```python
from build123d import *

# Parameters (mm, degrees)
F0_R     = 1.2
F0_W     = 10.5
F0_H     = 10.5
F1_DEPTH = 1.5
F2_DEPTH = 5.25
F3_DEPTH = 5.75
F5_DEPTH = 2


# Not quite as in the source:
# - a feature names something its author has since deleted; it is built from what else it names


with BuildPart() as f1:
    # F0 (on Top) → F1 (new body)
    with BuildSketch(Plane.XY):
        with BuildLine():
            Line((14.9310000289, -10.5), (14.9310000289, 10.5))
            ThreePointArc((14.9310000289, 10.5), (13.4665339264, 14.0355339264), (9.931, 15.5000000289))
            Line((9.931, 15.5000000289), (-9.931, 15.5000000289))
            ThreePointArc((-9.931, 15.5000000289), (-13.4665339264, 14.0355339264), (-14.9310000289, 10.5))
            Line((-14.9310000289, 10.5), (-14.9310000289, -10.5))
            ThreePointArc((-14.9310000289, -10.5), (-13.4665339264, -14.0355339264), (-9.931, -15.5000000289))
            Line((-9.931, -15.5000000289), (9.931, -15.5000000289))
            ThreePointArc((9.931, -15.5000000289), (13.4665339264, -14.0355339264), (14.9310000289, -10.5))
        make_face()
        with BuildLine():
            Line((-9.931, 13.5000000289), (-7.581, 13.5000000289))
            Line((-7.581, 13.5000000289), (0.069, 13.5000000289))
            Line((0.069, 13.5000000289), (4.769, 13.5000000289))
            Line((4.769, 13.5000000289), (9.931, 13.5000000289))
            ThreePointArc((9.931, 13.5000000289), (12.052320364, 12.621320364), (12.9310000289, 10.5))
            Line((12.9310000289, 10.5), (12.9310000289, -10.5))
            ThreePointArc((12.9310000289, -10.5), (12.052320364, -12.621320364), (9.931, -13.5000000289))
            Line((9.931, -13.5000000289), (4.769, -13.5000000289))
            Line((4.769, -13.5000000289), (0.069, -13.5000000289))
            Line((0.069, -13.5000000289), (-7.581, -13.5000000289))
            Line((-7.581, -13.5000000289), (-9.931, -13.5000000289))
            ThreePointArc((-9.931, -13.5000000289), (-12.052320364, -12.621320364), (-12.9310000289, -10.5))
            Line((-12.9310000289, -10.5), (-12.9310000289, -8.1))
            Line((-12.9310000289, -8.1), (-12.9310000289, 8.1))
            Line((-12.9310000289, 8.1), (-12.9310000289, 10.5))
            ThreePointArc((-12.9310000289, 10.5), (-12.052320364, 12.621320364), (-9.931, 13.5000000289))
        make_face(mode=Mode.SUBTRACT)
        with BuildLine():
            ThreePointArc((4.769, -10.45), (2.419, -8.1), (0.069, -10.45))
            ThreePointArc((0.069, -10.45), (2.419, -12.8), (4.769, -10.45))
        make_face()
        with Locations((2.419, -10.45)):
            Circle(F0_R, mode=Mode.SUBTRACT)
        with BuildLine():
            ThreePointArc((4.769, 10.45), (2.419, 12.8), (0.069, 10.45))
            ThreePointArc((0.069, 10.45), (2.419, 8.1), (4.769, 10.45))
        make_face()
        with Locations((2.419, 10.45)):
            Circle(F0_R, mode=Mode.SUBTRACT)
        with BuildLine():
            ThreePointArc((-9.931, 8.1), (-11.5927009358, 12.1117009358), (-7.581, 10.45))
            Line((-7.581, 10.45), (-7.581, 13.5000000289))
            Line((-7.581, 13.5000000289), (-9.931, 13.5000000289))
            ThreePointArc((-9.931, 13.5000000289), (-12.052320364, 12.621320364), (-12.9310000289, 10.5))
            Line((-12.9310000289, 10.5), (-12.9310000289, 8.1))
            Line((-12.9310000289, 8.1), (-9.931, 8.1))
        make_face()
        with BuildLine():
            Line((-9.931, -8.1), (-12.9310000289, -8.1))
            Line((-12.9310000289, -8.1), (-12.9310000289, -10.5))
            ThreePointArc((-12.9310000289, -10.5), (-12.052320364, -12.621320364), (-9.931, -13.5000000289))
            Line((-9.931, -13.5000000289), (-7.581, -13.5000000289))
            Line((-7.581, -13.5000000289), (-7.581, -10.45))
            ThreePointArc((-7.581, -10.45), (-11.5927009358, -12.1117009358), (-9.931, -8.1))
        make_face()
        with BuildLine():
            Line((-7.581, 13.5000000289), (-7.581, 10.45))
            ThreePointArc((-7.581, 10.45), (-8.2692990642, 8.7882990642), (-9.931, 8.1))
            Line((-9.931, 8.1), (-12.9310000289, 8.1))
            Line((-12.9310000289, 8.1), (-12.9310000289, -8.1))
            Line((-12.9310000289, -8.1), (-9.931, -8.1))
            ThreePointArc((-9.931, -8.1), (-8.2692990642, -8.7882990642), (-7.581, -10.45))
            Line((-7.581, -10.45), (-7.581, -13.5000000289))
            Line((-7.581, -13.5000000289), (0.069, -13.5000000289))
            Line((0.069, -13.5000000289), (0.069, -10.45))
            ThreePointArc((0.069, -10.45), (2.419, -8.1), (4.769, -10.45))
            Line((4.769, -10.45), (4.769, -13.5000000289))
            Line((4.769, -13.5000000289), (9.931, -13.5000000289))
            ThreePointArc((9.931, -13.5000000289), (12.052320364, -12.621320364), (12.9310000289, -10.5))
            Line((12.9310000289, -10.5), (12.9310000289, 10.5))
            ThreePointArc((12.9310000289, 10.5), (12.052320364, 12.621320364), (9.931, 13.5000000289))
            Line((9.931, 13.5000000289), (4.769, 13.5000000289))
            Line((4.769, 13.5000000289), (4.769, 10.45))
            ThreePointArc((4.769, 10.45), (2.419, 8.1), (0.069, 10.45))
            Line((0.069, 10.45), (0.069, 13.5000000289))
            Line((0.069, 13.5000000289), (-7.581, 13.5000000289))
        make_face()
        with Locations((2.469, 0)):
            Rectangle(F0_W, F0_H, mode=Mode.SUBTRACT)
        with BuildLine():
            ThreePointArc((-7.581, -10.45), (-8.2692990642, -8.7882990642), (-9.931, -8.1))
            ThreePointArc((-9.931, -8.1), (-11.5927009358, -12.1117009358), (-7.581, -10.45))
        make_face()
        with Locations((-9.931, -10.45)):
            Circle(F0_R, mode=Mode.SUBTRACT)
        with BuildLine():
            Line((0.069, -10.45), (0.069, -13.5000000289))
            Line((0.069, -13.5000000289), (4.769, -13.5000000289))
            Line((4.769, -13.5000000289), (4.769, -10.45))
            ThreePointArc((4.769, -10.45), (2.419, -12.8), (0.069, -10.45))
        make_face()
        with BuildLine():
            ThreePointArc((-9.931, 8.1), (-8.2692990642, 8.7882990642), (-7.581, 10.45))
            ThreePointArc((-7.581, 10.45), (-11.5927009358, 12.1117009358), (-9.931, 8.1))
        make_face()
        with Locations((-9.931, 10.45)):
            Circle(F0_R, mode=Mode.SUBTRACT)
        with BuildLine():
            Line((4.769, 13.5000000289), (0.069, 13.5000000289))
            Line((0.069, 13.5000000289), (0.069, 10.45))
            ThreePointArc((0.069, 10.45), (2.419, 12.8), (4.769, 10.45))
            Line((4.769, 10.45), (4.769, 13.5000000289))
        make_face()
    extrude(amount=F1_DEPTH)

    # F0 (on Top) → F2 (join)
    with BuildSketch(Plane.XY):
        with BuildLine():
            ThreePointArc((-9.931, 8.1), (-11.5927009358, 12.1117009358), (-7.581, 10.45))
            Line((-7.581, 10.45), (-7.581, 13.5000000289))
            Line((-7.581, 13.5000000289), (-9.931, 13.5000000289))
            ThreePointArc((-9.931, 13.5000000289), (-12.052320364, 12.621320364), (-12.9310000289, 10.5))
            Line((-12.9310000289, 10.5), (-12.9310000289, 8.1))
            Line((-12.9310000289, 8.1), (-9.931, 8.1))
        make_face()
        with BuildLine():
            ThreePointArc((-9.931, 8.1), (-8.2692990642, 8.7882990642), (-7.581, 10.45))
            ThreePointArc((-7.581, 10.45), (-11.5927009358, 12.1117009358), (-9.931, 8.1))
        make_face()
        with Locations((-9.931, 10.45)):
            Circle(F0_R, mode=Mode.SUBTRACT)
        with BuildLine():
            ThreePointArc((4.769, 10.45), (2.419, 12.8), (0.069, 10.45))
            ThreePointArc((0.069, 10.45), (2.419, 8.1), (4.769, 10.45))
        make_face()
        with Locations((2.419, 10.45)):
            Circle(F0_R, mode=Mode.SUBTRACT)
        with BuildLine():
            Line((4.769, 13.5000000289), (0.069, 13.5000000289))
            Line((0.069, 13.5000000289), (0.069, 10.45))
            ThreePointArc((0.069, 10.45), (2.419, 12.8), (4.769, 10.45))
            Line((4.769, 10.45), (4.769, 13.5000000289))
        make_face()
        with BuildLine():
            ThreePointArc((4.769, -10.45), (2.419, -8.1), (0.069, -10.45))
            ThreePointArc((0.069, -10.45), (2.419, -12.8), (4.769, -10.45))
        make_face()
        with Locations((2.419, -10.45)):
            Circle(F0_R, mode=Mode.SUBTRACT)
        with BuildLine():
            Line((0.069, -10.45), (0.069, -13.5000000289))
            Line((0.069, -13.5000000289), (4.769, -13.5000000289))
            Line((4.769, -13.5000000289), (4.769, -10.45))
            ThreePointArc((4.769, -10.45), (2.419, -12.8), (0.069, -10.45))
        make_face()
        with BuildLine():
            ThreePointArc((-7.581, -10.45), (-8.2692990642, -8.7882990642), (-9.931, -8.1))
            ThreePointArc((-9.931, -8.1), (-11.5927009358, -12.1117009358), (-7.581, -10.45))
        make_face()
        with Locations((-9.931, -10.45)):
            Circle(F0_R, mode=Mode.SUBTRACT)
        with BuildLine():
            Line((-9.931, -8.1), (-12.9310000289, -8.1))
            Line((-12.9310000289, -8.1), (-12.9310000289, -10.5))
            ThreePointArc((-12.9310000289, -10.5), (-12.052320364, -12.621320364), (-9.931, -13.5000000289))
            Line((-9.931, -13.5000000289), (-7.581, -13.5000000289))
            Line((-7.581, -13.5000000289), (-7.581, -10.45))
            ThreePointArc((-7.581, -10.45), (-11.5927009358, -12.1117009358), (-9.931, -8.1))
        make_face()
    extrude(amount=F2_DEPTH)

    # F0 (on Top) → F3 (join)
    with BuildSketch(Plane.XY):
        with BuildLine():
            Line((14.9310000289, -10.5), (14.9310000289, 10.5))
            ThreePointArc((14.9310000289, 10.5), (13.4665339264, 14.0355339264), (9.931, 15.5000000289))
            Line((9.931, 15.5000000289), (-9.931, 15.5000000289))
            ThreePointArc((-9.931, 15.5000000289), (-13.4665339264, 14.0355339264), (-14.9310000289, 10.5))
            Line((-14.9310000289, 10.5), (-14.9310000289, -10.5))
            ThreePointArc((-14.9310000289, -10.5), (-13.4665339264, -14.0355339264), (-9.931, -15.5000000289))
            Line((-9.931, -15.5000000289), (9.931, -15.5000000289))
            ThreePointArc((9.931, -15.5000000289), (13.4665339264, -14.0355339264), (14.9310000289, -10.5))
        make_face()
        with BuildLine():
            Line((-9.931, 13.5000000289), (-7.581, 13.5000000289))
            Line((-7.581, 13.5000000289), (0.069, 13.5000000289))
            Line((0.069, 13.5000000289), (4.769, 13.5000000289))
            Line((4.769, 13.5000000289), (9.931, 13.5000000289))
            ThreePointArc((9.931, 13.5000000289), (12.052320364, 12.621320364), (12.9310000289, 10.5))
            Line((12.9310000289, 10.5), (12.9310000289, -10.5))
            ThreePointArc((12.9310000289, -10.5), (12.052320364, -12.621320364), (9.931, -13.5000000289))
            Line((9.931, -13.5000000289), (4.769, -13.5000000289))
            Line((4.769, -13.5000000289), (0.069, -13.5000000289))
            Line((0.069, -13.5000000289), (-7.581, -13.5000000289))
            Line((-7.581, -13.5000000289), (-9.931, -13.5000000289))
            ThreePointArc((-9.931, -13.5000000289), (-12.052320364, -12.621320364), (-12.9310000289, -10.5))
            Line((-12.9310000289, -10.5), (-12.9310000289, -8.1))
            Line((-12.9310000289, -8.1), (-12.9310000289, 8.1))
            Line((-12.9310000289, 8.1), (-12.9310000289, 10.5))
            ThreePointArc((-12.9310000289, 10.5), (-12.052320364, 12.621320364), (-9.931, 13.5000000289))
        make_face(mode=Mode.SUBTRACT)
    extrude(amount=F3_DEPTH)

    # F4 (on face) → F5 (cut)
    with BuildSketch(Plane(origin=(-14.9310000289, 0, 0), x_dir=(0, -1, 0), z_dir=(-1, 0, 0))):
        with BuildLine():
            Line((7, 5.75), (-7, 5.75))
            Line((-7, 5.75), (-7, 5))
            ThreePointArc((-7, 5), (-6.8535533906, 4.6464466094), (-6.5, 4.5))
            Line((-6.5, 4.5), (6.5, 4.5))
            ThreePointArc((6.5, 4.5), (6.8535533906, 4.6464466094), (7, 5))
            Line((7, 5), (7, 5.75))
        make_face()
    extrude(amount=-F5_DEPTH, mode=Mode.SUBTRACT)


solid = f1.part
```
Can you work these out from the model? Positions are in its coordinate system, mm. A direction names the side the tool comes from. Round coordinates to 2 decimals unless told otherwise and drop trailing zeros. Order: outer loops, then holes, each group sorted by start corner. A loop starts at its lowest first (then second) coordinate and runs counter-clockwise, first axis right, second up. Notation, with made-up numbers: (15, 10.25) -> (48, 10.25) arc R10 ccw to (48, 15.25) -> close; hole circle Ø8 at (79.25, 12.5). An arc over 180 degrees is marked (long way). Return JSON: item names as keys, results as strings. Group by question number.
1. If we section it at D-D, the plane z = 2.7: Count the separate pieces of the cut face and the enclosed holes in it, then the cut area to 3 significant figures.
2. We'd pull the mould along X, two halves only. Please class faces 5 (the face through (2, -12, 5.25)), 6 (the face through (0, 15.5, 3)), 7 (the face through (-14.931, 0, 2)): released by +X, released by -X, zero draft, split by the parting line, or undercut.
3. I need wall thicknesses on line 1 (Y direction, x = 2.5, z = 4.15); line 2 (Y direction, x = 6.5, z = 4.2); line 3 (X direction, y = -9.5, z = 1.25). Which ranges of each line are inside material? Lowest first, please. Write a range as [from, to].
4. If we section it at A-A, the plane y = -2: Write out the boundary of the cut face in (x, z), then the cut area to 3 significant figures.
5. If we section it at B-B, the plane z = 0.7: Write out the boundary of the cut face in (x, y), then the cut area to 3 significant figures.
6. Will these pins go through, and if not, where does the flat tip stop? pin 1 (0.9 mm diameter, centred on x = -11.5, z = 4, fed in from -Y); pin 2 (5 mm diameter, centred on x = 1.5, y = -10, fed in from +Z); pin 3 (10 mm diameter, centred on x = 10.5, y = 5, fed in from +Z); pin 4 (1.5 mm diameter, centred on y = 11.5, z = 3.5, fed in from +X).
7. Which directions (+Z, -Z, +X, -X, +Y, -Y) give clear straight access to the entire face, cutting with the end or side of a thin tool? Please do faces 1 (the face through (-14, 0, 4.5)), 2 (the face through (-4, 0, 0)), 3 (the face through (2, -5.25, 1)), 4 (the face through (0.069, 12, 3)).
8. If we section it at C-C, the plane x = 9.5: Write out the boundary of the cut face in (y, z), then the cut area to 3 significant figures.
Output values:
{
 "1": {"separate pieces": "1", "enclosed holes": "5", "area": "293 mm²"},
 "2": {"face 5": "undercut", "face 6": "zero draft", "face 7": "released by -X"},
 "3": {"line 1": "[-15.5, -11.65], [-9.25, -8.1], [8.1, 9.25], [11.65, 15.5]", "line 2": "[-15.5, -13.5], [13.5, 15.5]", "line 3": "[-14.93, -10.66], [-9.2, 1.69], [3.15, 14.93]"},
 "4": {"outline": "(-14.93, 0) -> (-2.78, 0) -> (-2.78, 1.5) -> (-12.93, 1.5) -> (-12.93, 4.5) -> (-14.93, 4.5) -> close; (7.72, 0) -> (14.93, 0) -> (14.93, 5.75) -> (12.93, 5.75) -> (12.93, 1.5) -> (7.72, 1.5) -> close", "area": "43.5 mm²"},
 "5": {"outline": "(-14.93, -10.5) arc R5 ccw to (-9.93, -15.5) -> (9.93, -15.5) arc R5 ccw to (14.93, -10.5) -> (14.93, 10.5) arc R5 ccw to (9.93, 15.5) -> (-9.93, 15.5) arc R5 ccw to (-14.93, 10.5) -> close; hole circle Ø2.4 at (-9.93, -10.45); hole circle Ø2.4 at (-9.93, 10.45); hole (-2.78, -5.25) -> (7.72, -5.25) -> (7.72, 5.25) -> (-2.78, 5.25) -> close; hole circle Ø2.4 at (2.42, -10.45); hole circle Ø2.4 at (2.42, 10.45)", "area": "776 mm²"},
 "6": {"pin 1": "y = -15.37", "pin 2": "z = 5.25", "pin 3": "z = 5.75", "pin 4": "x = 14.92"},
 "7": {"face 1": "+Z, -X", "face 2": "-Z, +X, -X, +Y, -Y", "face 3": "+Z, -Z", "face 4": "+Z"},
 "8": {"outline": "(-15.5, 0) -> (15.5, 0) -> (15.5, 5.75) -> (13.5, 5.75) -> (13.5, 1.5) -> (-13.5, 1.5) -> (-13.5, 5.75) -> (-15.5, 5.75) -> close", "area": "63.5 mm²"}
}
